Read the model definition and answer for the solid it produces. Units are mm, in the model's axes. Coordinates: 2 decimals unless noted, no trailing zeros. Write each loop counter-clockwise with the first axis right and the second up, starting at its lowest first coordinate (ties: lowest second). Pieces come first, ordered by that corner, then holes. Notation, with made-up numbers: (15.5, -22) -> (31.5, -22) arc R18 ccw to (31.5, 13) -> close; hole circle Ø3 at (60.25, 80.5). An arc over 180 degrees is marked (long way). Write item = value, one per line. Start each with the question number.
1) Find the intervals of material crossed by line 1 along Y through (x, z) = (15.5, 1.75); line 2 along X through (y, z) = (-27, 7) (3 decimals); line 3 along Y through (x, z) = (-2, 14), in increasing order. Write a range as from..to.
2) Section D-D (z = 29.5) is taken. Determine the outline of the cut face in (x, y), plus the area to 3 significant figures.
3) Flat-ended cylindrical pins translate along their axes: pin 1 Ø4 at (x, y) = (9, 8.5) entering from +Z; pin 2 Ø2 at (x, z) = (-1, 30) entering from +Y; pin 3 Ø3.5 at (x, z) = (-19.375, 38) entering from -Y. Find the tip coordinate at first contact, or state that the pin passes through.
4) Section C-C (z = 7) is taken. Determine the outline of the cut face in (x, y) (1 decimal).
5) Section B-B (y = -15.5) is taken. Determine the outline of the cut face in (x, z), plus the area to 3 significant figures.
6) Section A-A (x = 15.5) is taken. Determine the outline of the cut face in (y, z), plus the area to 4 significant figures.
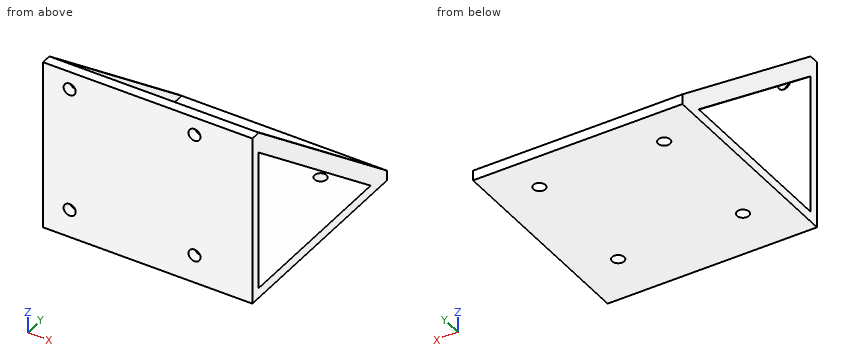
from build123d import *

# Parameters (mm, degrees)
SKETCH1_R           = 1.5
BOSS_EXTRUDE1_DEPTH = 2.5
SKETCH2_W           = 50
SKETCH2_H           = 2.5
BOSS_EXTRUDE2_DEPTH = 40
SKETCH3_R           = 1.5
CUT_EXTRUDE1_DEPTH  = 40
BOSS_EXTRUDE3_DEPTH = 1


with BuildPart() as part:
    # Sketch1 → Boss-Extrude1 (new body)
    with BuildSketch(Plane.XY):
        Polygon((-25, -25), (-25, 25), (25, 25), (25, -25), (25, -28), (-25, -28), align=None)
        with Locations((-15.5, 15.5)):
            Circle(SKETCH1_R, mode=Mode.SUBTRACT)
        with Locations((15.5, 15.5)):
            Circle(SKETCH1_R, mode=Mode.SUBTRACT)
        with Locations((15.5, -15.5)):
            Circle(SKETCH1_R, mode=Mode.SUBTRACT)
        with Locations((-15.5, -15.5)):
            Circle(SKETCH1_R, mode=Mode.SUBTRACT)
    extrude(amount=BOSS_EXTRUDE1_DEPTH)

    # Sketch2 → Boss-Extrude2 (add)
    with BuildSketch(Plane.XY.offset(2.5)):
        with Locations((0, -26.75)):
            Rectangle(SKETCH2_W, SKETCH2_H)
    extrude(amount=BOSS_EXTRUDE2_DEPTH)

    # Sketch3 → Cut-Extrude1 (cut)
    with BuildSketch(Plane(origin=(0, -25.5, 0), x_dir=(1, 0, 0), z_dir=(0, 1, 0))):
        with Locations((-19.375, -7)):
            Circle(SKETCH3_R)
        with Locations((11.625, -7)):
            Circle(SKETCH3_R)
        with Locations((11.625, -38)):
            Circle(SKETCH3_R)
        with Locations((-19.375, -38)):
            Circle(SKETCH3_R)
    extrude(amount=-CUT_EXTRUDE1_DEPTH, mode=Mode.SUBTRACT)

    # Sketch5 → Boss-Extrude3 (add)
    with BuildSketch(Plane(origin=(25, 0, 0), x_dir=(0, 0, -1), z_dir=(1, 0, 0))):
        Polygon((-42.5, -25.5), (-2.5, 25), (0, 25), (0, 16.843145751), (0, -28), (-39.343145751, -28), (-42.5, -28), align=None)
        Polygon((-2.5, 18.557756602), (-37.397232952, -25.5), (-2.5, -25.5), align=None, mode=Mode.SUBTRACT)
    boss_extrude3 = extrude(amount=BOSS_EXTRUDE3_DEPTH)

    # Mirror1: Boss-Extrude3 across plane
    add(boss_extrude3.mirror(Plane(origin=(0, 0, 0), x_dir=(0, 0, 1), z_dir=(1, 0, 0))))


solid = part.part
Answer key:
q1.line_1 = -28..-17, -14..14, 17..25
q1.line_2 = -26..-20.875, -17.875..10.125, 13.125..26
q1.line_3 = -28..-25.5
q2.outline = (-26, -28) -> (26, -28) -> (26, -25.5) -> (-26, -25.5) -> close; (-26, -15.53) -> (-25, -15.53) -> (-25, -9.09) -> (-26, -9.09) -> close; (25, -15.53) -> (26, -15.53) -> (26, -9.09) -> (25, -9.09) -> close
q2.area = 143 mm^2
q3.pin_1 = 2.5
q3.pin_2 = -25.5
q3.pin_3 = -28
q4.outline = (-26, -28) -> (-20.9, -28) -> (-20.9, -25.5) -> (-26, -25.5) -> close; (-26, 12.9) -> (-25, 12.9) -> (-25, 19.3) -> (-26, 19.3) -> close; (-17.9, -28) -> (10.1, -28) -> (10.1, -25.5) -> (-17.9, -25.5) -> close; (13.1, -28) -> (26, -28) -> (26, -25.5) -> (13.1, -25.5) -> close; (25, 12.9) -> (26, 12.9) -> (26, 19.3) -> (25, 19.3) -> close
q5.outline = (-26, 0) -> (-17, 0) -> (-17, 2.5) -> (-26, 2.5) -> close; (-26, 29.48) -> (-25, 29.48) -> (-25, 34.58) -> (-26, 34.58) -> close; (-14, 0) -> (14, 0) -> (14, 2.5) -> (-14, 2.5) -> close; (17, 0) -> (26, 0) -> (26, 2.5) -> (17, 2.5) -> close; (25, 29.48) -> (26, 29.48) -> (26, 34.58) -> (25, 34.58) -> close
q5.area = 125 mm^2
q6.outline = (-28, 0) -> (-17, 0) -> (-17, 2.5) -> (-25.5, 2.5) -> (-25.5, 42.5) -> (-28, 42.5) -> close; (-14, 0) -> (14, 0) -> (14, 2.5) -> (-14, 2.5) -> close; (17, 0) -> (25, 0) -> (25, 2.5) -> (17, 2.5) -> close
q6.area = 217.5 mm^2
